For this review, take the finished solid that the model builds, in its own axes (mm). A direction names the side the tool comes from. Coordinates: 2 decimals unless noted, no trailing zeros. Order: outer loops, then holes, each group sorted by start corner. A loop starts at its lowest first (then second) coordinate and runs counter-clockwise, first axis right, second up. Notation, with made-up numbers: (17.25, 31.25) -> (53.25, 31.25) arc R13 ccw to (53.25, 35.25) -> close; hole circle Ø8 at (61, 0). An arc over 180 degrees is marked (long way). Write item = value, one per line. Start each with the question number.
1) Consider section B-B on x = -3. Give the boundary of the cut face in (y, z).
2) Consider section D-D on x = 23. Give the boundary of the cut face in (y, z), and give its area (3 significant figures).
3) Wall thickness on probe 1 along Z at (x, y) = (2, -2.75); probe 2 along Z at (x, y) = (-28, -7.25); probe 3 along Z at (x, y) = (25.5, -1): over which ranges is each line inside the solid? List them lowest first. Write a range as [from, to].
4) Machinability: for faces 5 (the face through (-12.72, -4.93, -23.145)), 6 (the face through (13.505, -4.93, 22.293)), 7 (the face through (-13.684, -4.93, 22.589)), which of the approach directions +Z, -Z, +X, -X, +Y, -Y give a long, thin tool a straight path to every point of the face, cutting with its end or side? Answer none if there is none.
5) Draft analysis for pull direction X (two halves, no side actions). For faces 1 (the face through (9.95, -4.93, 9.67)), 2 (the face through (-9.88, -4.93, 9.74)), 3 (the face through (26.42, -4.93, -26.27)), 4 (the face through (-1.3, -4.93, 42.93)), state which applies: +X half, -X half, draft (parallel to the pull), parting line (faces both ways), or undercut.
6) Insertion check: pin 1 Ø1 at (x, y) = (-5.5, -5.5) entering from -Z; pin 2 Ø10 at (x, z) = (-2, -2) entering from +Y; pin 3 Ø1 at (y, z) = (-6.5, 7.5) entering from +X; pin 4 Ø1.5 at (y, z) = (-8, 12.5) entering from -X. Each pin has a flat end and moves straight along its axis. Give the tip position at first contact, or say it passes through.
7) Consider section C-C on y = -5.5. Give the boundary of the cut face in (x, z).
8) Consider section A-A on x = 33. Give the boundary of the cut face in (y, z).
from build123d import *

# Parameters (mm, degrees)
F0_R     = 10
F1_DEPTH = 10


with BuildPart() as f1:
    # F0 (on Front) → F1 (new body)
    with BuildSketch(Plane.XZ):
        with BuildLine():
            Line((-20, 33.013921), (-7.189306, 11.86736))
            ThreePointArc((-7.189306, 11.86736), (-9.914082, 9.707283), (-12.01625, 6.937585))
            ThreePointArc((-12.01625, 6.937585), (-13.363794, 3.732205), (-13.872088, 0.292442))
            Line((-13.872088, 0.292442), (-38.590894, 0.813547))
            ThreePointArc((-38.590894, 0.813547), (-45.509288, -11.215099), (-43.092199, -24.879293))
            ThreePointArc((-43.092199, -24.879293), (-32.467205, -33.80465), (-18.590894, -33.827469))
            Line((-18.590894, -33.827469), (-6.682782, -12.159802))
            ThreePointArc((-6.682782, -12.159802), (-3.449712, -13.439488), (0, -13.87517))
            ThreePointArc((0, -13.87517), (3.449712, -13.439488), (6.682782, -12.159802))
            Line((6.682782, -12.159802), (18.590894, -33.827469))
            ThreePointArc((18.590894, -33.827469), (32.467205, -33.80465), (43.092199, -24.879293))
            ThreePointArc((43.092199, -24.879293), (45.509288, -11.215099), (38.590894, 0.813547))
            Line((38.590894, 0.813547), (13.872088, 0.292442))
            ThreePointArc((13.872088, 0.292442), (13.363794, 3.732205), (12.01625, 6.937585))
            ThreePointArc((12.01625, 6.937585), (9.914082, 9.707283), (7.189306, 11.86736))
            Line((7.189306, 11.86736), (20, 33.013921))
            ThreePointArc((20, 33.013921), (13.042084, 45.019749), (0, 49.758585))
            ThreePointArc((0, 49.758585), (-13.042084, 45.019749), (-20, 33.013921))
        make_face()
        with Locations((-28.590894, -16.506961)):
            Circle(F0_R, mode=Mode.SUBTRACT)
        with Locations((28.590894, -16.506961)):
            Circle(F0_R, mode=Mode.SUBTRACT)
        with BuildLine():
            ThreePointArc((-9.526279, 5.5), (0, 11), (9.526279, 5.5))
            ThreePointArc((9.526279, 5.5), (9.526279, -5.5), (0, -11))
            ThreePointArc((0, -11), (-9.526279, -5.5), (-9.526279, 5.5))
        make_face(mode=Mode.SUBTRACT)
        with Locations((0, 33.013921)):
            Circle(F0_R, mode=Mode.SUBTRACT)
    extrude(amount=F1_DEPTH)


solid = f1.part
Answer sheet:
q1.outline = (-10, -13.55) -> (0, -13.55) -> (0, -10.58) -> (-10, -10.58) -> close; (-10, 10.58) -> (0, 10.58) -> (0, 23.47) -> (-10, 23.47) -> close; (-10, 42.55) -> (0, 42.55) -> (0, 49.54) -> (-10, 49.54) -> close
q2.outline = (-10, -34.88) -> (0, -34.88) -> (0, -24.8) -> (-10, -24.8) -> close; (-10, -8.22) -> (0, -8.22) -> (0, 0.48) -> (-10, 0.48) -> close
q2.area = 188 mm2
q3.probe_1 = [-13.73, -10.82], [10.82, 23.22], [42.81, 49.66]
q3.probe_2 = [-34.88, -26.49], [-6.52, 0.59]
q3.probe_3 = [-35.04, -26.02], [-7, 0.54]
q4.face_5 = -Z, +Y, -Y
q4.face_6 = +X, +Y, -Y
q4.face_7 = -X, +Y, -Y
q5.face_1 = +X half
q5.face_2 = -X half
q5.face_3 = undercut
q5.face_4 = undercut
q6.pin_1 = -12.94
q6.pin_2 = through
q6.pin_3 = 11.98
q6.pin_4 = -8.03
q7.outline = (-43.09, -24.88) arc R20.32 ccw to (-18.59, -33.83) -> (-6.68, -12.16) arc R13.88 ccw to (0, -13.88) arc R13.88 ccw to (6.68, -12.16) -> (18.59, -33.83) arc R20.32 ccw to (43.09, -24.88) arc R20.32 ccw to (38.59, 0.81) -> (13.87, 0.29) arc R13.88 ccw to (12.02, 6.94) arc R13.88 ccw to (7.19, 11.87) -> (20, 33.01) arc R20.32 ccw to (0, 49.76) arc R20.32 ccw to (-20, 33.01) -> (-7.19, 11.87) arc R13.88 ccw to (-12.02, 6.94) arc R13.88 ccw to (-13.87, 0.29) -> (-38.59, 0.81) arc R20.32 ccw to start; hole circle Ø20 at (-28.59, -16.51); hole circle Ø22 at (0, 0); hole circle Ø20 at (0, 33.01); hole circle Ø20 at (28.59, -16.51)
q8.outline = (-10, -33.6) -> (0, -33.6) -> (0, -25.48) -> (-10, -25.48) -> close; (-10, -7.53) -> (0, -7.53) -> (0, 0.7) -> (-10, 0.7) -> close
